The model under review builds one solid part; all positions refer to its coordinate system, in mm. Face numbers are marked on the shaded views. Coordinates: 2 decimals unless noted, no trailing zeros. Loops run counter-clockwise (first coordinate to the right, second up) from the corner with the lowest first, then second, coordinate; pieces in that order, holes last. Notation, with made-up numbers: M -1,-20 L 32,-20 A22 cw 32,15 Z; hole C 65.25,-30.5 d8. An arc over 180 degrees is marked long. Use CSV: the item, a comma, the result in double quotes. Start each with the question number.
1. Clearance check with a flat-ended pin moving along its axis: P1, Ø4, axis at x = -4.5, z = 6, coming from the +Y side. State where the tip first meets the part, or that it passes through.
2. Add section B-B, the plane z = 6.5. Write out the cut boundary in (x, y), then the cut area to 3 significant figures.
3. For L1, parallel to X at y = 0, z = 5.5; L2, parallel to Z at x = -2.75, y = 4.5, list the stretches that pass through material, from the lowest coordinate up.
4. Add section A-A, the plane x = 0. Write out the cut boundary in (y, z).
5. Draft analysis for pull direction X (two halves, no side actions). For the marked faces 1, 2 and 3, state which applies: +X half, -X half, draft (parallel to the pull), parting line (faces both ways), or undercut.
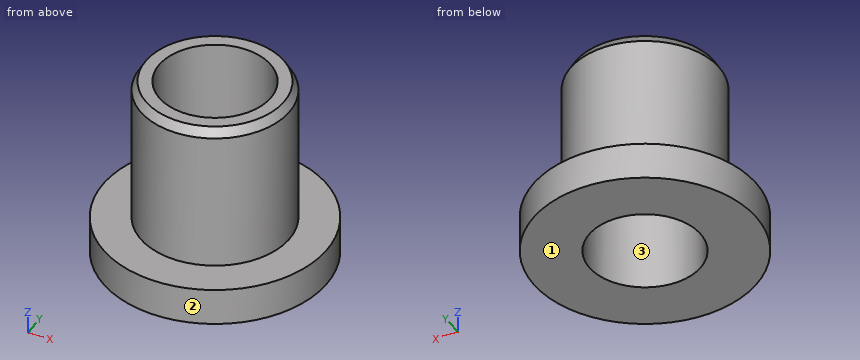
Autodesk Inventor part; units mm, degrees
ref_plane "YZ Plane" through (0, 0, 0) normal (1, 0, 0) x (0, 1, 0)
ref_plane "XZ Plane" through (0, 0, 0) normal (0, 1, 0) x (-1, 0, 0)
ref_plane "XY Plane" through (0, 0, 0) normal (0, 0, 1) x (1, 0, 0)
sketch "Sketch1" plane through (0, 0, 0) normal (0, 0, 1) x (1, 0, 0)
  circle A0 centre (0, 0) radius 6
  circle A1 centre (0, 0) radius 3 construction
  circle A2 centre (0, 0) radius 4
  dimension "dia_Flange" = 12
  dimension "dia_Shaft" = 6
  dimension "dia_Outer" = 8
extrude "Extrusion1" add sketch "Sketch1" along normal blind 2 contours A0 | A2
extrude "Extrusion2" add sketch "Sketch1" along normal blind 10 contours A2
chamfer "Chamfer1" distance 0.5 angle 30 1 edges at (-4, 0, 10) measured on face at (3.9482, 0.6416, 4.6667)
hole "Hole1" at (0, 0, 0) direction (0, 0, 1) diameter 6 end through all
equation "\"d10\" = dia_Shaft"
properties part number "GFM-0608-10_Brass" material "Brass"
Computed:
1,P1,"stops at y = 3.12"
2,outline,"C 0,0 d8; hole C 0,0 d6"
2,area,"22.0 mm^2"
3,L1,"x = -4 to -3, 3 to 4"
3,L2,"z = 0 to 2"
4,outline,"M -6,0 L -3,0 L -3,10 L -3.71,10 L -4,9.5 L -4,2 L -6,2 Z; M 3,0 L 6,0 L 6,2 L 4,2 L 4,9.5 L 3.71,10 L 3,10 Z"
5,face 1,"draft"
5,face 2,"parting line"
5,face 3,"undercut"
